For this review, take the finished solid that the model builds, in its own axes (mm). Round coordinates to 2 decimals unless told otherwise and drop trailing zeros. Loops run counter-clockwise (first coordinate to the right, second up) from the corner with the lowest first, then second, coordinate; pieces in that order, holes last.
1. Consider section D-D on z = -74. State the section outline as (x, y) points.
2. Clearance check with flat-ended pins moving along their axes: pin 1 Ø5 at (x, y) = (31, -4) entering from -Z; pin 2 Ø5 at (x, y) = (36.5, -5) entering from +Z; pin 3 Ø4 at (x, y) = (-38.5, -5.5) entering from -Z. State where each tip first meets the part, or that it passes through.
3. Consider section A-A on z = 0. State the section outline as (x, y) points.
4. To check wall thickness, follow line 1 along X through (y, z) = (-5.25, 0); line 2 along Z through (x, y) = (2, -6); line 3 along X through (y, z) = (-8, -49). State the ranges of each line that lie inside material, in increasing order.
5. Consider section C-C on x = 0. State the section outline as (y, z) points.
6. Consider section B-B on y = -6.5. State the section outline as (x, z) points.
from build123d import *

# Parameters (mm, degrees)
F0_R     = 8
F1_DEPTH = 9.2


with BuildPart() as f1:
    # F0 (on Front) → F1 (new body)
    with BuildSketch(Plane.XZ):
        with BuildLine():
            Line((76.2651364849, -104.9699550201), (99.9234928897, -137.5328890437))
            ThreePointArc((99.9234928897, -137.5328890437), (5.9329144394, 169.8964405932), (-109.2738936467, -130.2275553302))
            Line((-109.2738936467, -130.2275553302), (-99.8627523041, -137.4492867999))
            Line((-99.8627523041, -137.4492867999), (-76.2651364849, -104.9699550201))
            ThreePointArc((-76.2651364849, -104.9699550201), (-10.7051286377, 129.3076282392), (92.4890377243, -90.9991230773))
            ThreePointArc((92.4890377243, -90.9991230773), (84.6657478828, -98.3197520107), (76.2651364849, -104.9699550201))
        make_face()
        with Locations((-128.1717597601, -74)):
            Circle(F0_R, mode=Mode.SUBTRACT)
        with Locations((128.1717597601, -74)):
            Circle(F0_R, mode=Mode.SUBTRACT)
        with Locations((0, 148)):
            Circle(F0_R, mode=Mode.SUBTRACT)
    extrude(amount=F1_DEPTH)


solid = f1.part
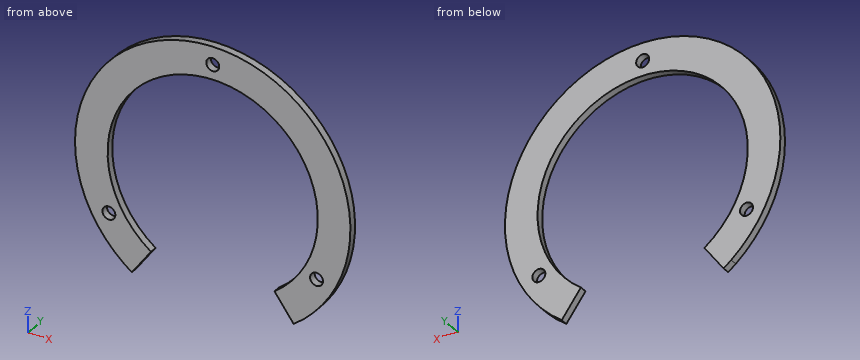
Resolved:
1. outline: (-153.05, -9.2) - (-136.17, -9.2) - (-136.17, 0) - (-153.05, 0) - close; (-120.17, -9.2) - (-106.58, -9.2) - (-106.58, 0) - (-120.17, 0) - close; (106.58, -9.2) - (120.17, -9.2) - (120.17, 0) - (106.58, 0) - close; (136.17, -9.2) - (153.05, -9.2) - (153.05, 0) - (136.17, 0) - close
2. pin 1: stops at z = 125.35
2. pin 2: stops at z = 166.57
2. pin 3: stops at z = 123.27
3. outline: (-170, -9.2) - (-129.75, -9.2) - (-129.75, 0) - (-170, 0) - close; (129.75, -9.2) - (170, -9.2) - (170, 0) - (129.75, 0) - close
4. line 1: x = -170 to -129.75, 129.75 to 170
4. line 2: z = 129.73 to 140.25, 155.75 to 169.99
4. line 3: x = -162.79 to -120.14, 120.14 to 162.79
5. outline: (-9.2, 129.75) - (0, 129.75) - (0, 140) - (-9.2, 140) - close; (-9.2, 156) - (0, 156) - (0, 170) - (-9.2, 170) - close
6. outline: (-109.27, -130.23) - (-99.86, -137.45) - (-76.27, -104.97) arc R129.75 cw (long way) to (76.27, -104.97) - (99.92, -137.53) arc R170 ccw (long way) to start; hole circle Ø16 at (-128.17, -74); hole circle Ø16 at (0, 148); hole circle Ø16 at (128.17, -74)
